Check sheet for the modelled part. Datum: model origin and axes. Units: mm. A direction names the side the tool comes from. Round coordinates to 2 decimals unless told otherwise and drop trailing zeros. Write each loop counter-clockwise with the first axis right and the second up, starting at its lowest first coordinate (ties: lowest second). Pieces come first, ordered by that corner, then holes.
Item 1: Tool access check on faces 1 (the flat face through (3.092, -9, 0.6)), 2 (the flat face through (0, -1, 1.118)). Record the directions out of +Z, -Z, +X, -X, +Y, -Y that give a thin tool (end or side, any length) a straight path to the whole face; none if there is none.
Item 2: Cross-section at C-C on x = 14.5. Enter the section's corners in (y, z), plus the area to 3 significant figures.
Item 3: Cross-section at A-A on z = 0.45. Enter the section's corners in (x, y).
Item 4: Material ranges on line 1 (X direction, y = -12, z = 0.65); line 2 (Y direction, x = 16, z = 0.55); line 3 (Y direction, x = 18.5, z = 0.8), recorded low to high.
Item 5: Cross-section at B-B on y = -16.5. Enter the section's corners in (x, z), plus the area to 3 significant figures.
Item 6: Release check for a two-part mould opening along X. For faces 3 (the flat face through (-3.279, -8.7, 0.6)), 4 (the flat face through (-20.325, -2.846, 0.551)), 5 (the flat face through (0, -1, 0)), 6 (the flat face through (-11.333, -2.664, 0.551)) record: +X half, -X half, draft (parallel to the pull), parting line (faces both ways), or undercut.
from build123d import *

# Parameters (mm, degrees)
F1_DEPTH = 1.1176


with BuildPart() as f1:
    # F0 (on Top) → F1 (new body)
    with BuildSketch(Plane.XY):
        Polygon((-3.279098, 0.532189), (-3.279098, 7.214016), (-21.454671, 0), (-19.16354, -5.77246), align=None)
        Polygon((3.091722, 7.214016), (-3.279098, 7.214016), (-3.279098, 0.532189), (-3.279098, -18.269263), (3.091722, -18.269263), (3.091722, 0.532189), align=None)
        Polygon((21.079501, -0.577142), (3.091722, 7.214016), (3.091722, 0.532189), (18.829221, -5.77246), align=None)
    extrude(amount=F1_DEPTH)


solid = f1.part
Response values:
1. face 1: +Z, -Z, -Y
1. face 2: +Z, +X, -X, +Y, -Y
2. outline: (-4.04, 0) - (2.27, 0) - (2.27, 1.12) - (-4.04, 1.12) - close
2. area: 7.05 mm2
3. outline: (-21.45, 0) - (-19.16, -5.77) - (-3.28, 0.53) - (-3.28, -18.27) - (3.09, -18.27) - (3.09, 0.53) - (18.83, -5.77) - (21.08, -0.58) - (3.09, 7.21) - (-3.28, 7.21) - close
4. line 1: x = -3.28 to 3.09
4. line 2: y = -4.64 to 1.62
4. line 3: y = -5.64 to 0.54
5. outline: (-3.28, 0) - (3.09, 0) - (3.09, 1.12) - (-3.28, 1.12) - close
5. area: 7.12 mm2
6. face 3: undercut
6. face 4: -X half
6. face 5: draft
6. face 6: undercut
